Work out the finished part from the listing and answer in its coordinate system (mm). Face numbers are marked on the shaded views. Give positions to 0.01 mm unless a question says otherwise; leave off trailing zeros. Write each loop counter-clockwise with the first axis right and the second up, starting at its lowest first coordinate (ties: lowest second). Pieces come first, ordered by that corner, then holes. Notation, with made-up numbers: (5.5, 19.5) -> (45.5, 19.5) arc R36 cw to (45.5, 56.5) -> close; hole circle Ø6 at (-20.75, -6.5). An arc over 180 degrees is marked (long way). Use a Markdown table: item, result. Add a question column.
Q1. Each of these flat-tipped pins is pushed along its axis until it touches: pin 1 Ø3 at (x, z) = (0, 0) entering from +Y; pin 2 Ø4.5 at (x, z) = (0, 0.5) entering from -Y; pin 3 Ø1 at (x, y) = (39, 0.5) entering from +Z; pin 4 Ø1 at (y, z) = (1, 24) entering from +X. Where does it stop, or does it pass through?
Q2. Section C-C, the plane z = 30 is taken. Give the vertices of the cut face in (x, y), plus the area to 3 significant figures.
Q3. Consider line 1 (X direction, y = 2.55, z = 0); line 2 (X direction, y = 1.15, z = 0); line 3 (X direction, y = 0.35, z = 0). Determine where each line is inside the solid, lowest interval first.
Q4. Section D-D, the plane x = 94.5 is taken. Give the vertices of the cut face in (y, z), plus the area to 3 significant figures.
Q5. Section B-B, the plane x = 52.5 is taken. Give the vertices of the cut face in (y, z), plus the area to 3 significant figures.
Q6. For a pull along Z with two mould halves and no side action, classify the marked faces 1 and 2 as pulls with the +Z half, pulls with the -Z half, needs draft (parallel to the pull), parting line crosses it, or undercut.
Q7. Section A-A, the plane z = 9.5 is taken. Give the vertices of the cut face in (x, y).
Autodesk Inventor part; units mm, degrees
ref_plane "YZ Plane" through (0, 0, 0) normal (1, 0, 0) x (0, 1, 0)
ref_plane "XZ Plane" through (0, 0, 0) normal (0, 1, 0) x (-1, 0, 0)
ref_plane "XY Plane" through (0, 0, 0) normal (0, 0, 1) x (1, 0, 0)
sketch "Szkic4" plane through (0, 0, 0) normal (0, 1, 0) x (-1, 0, 0)
  circle A0 centre (0, 0) radius 2.1
  line L0 (-3, 3) -> (3, 3)
  line L1 (3, 3) -> (3, -3)
  line L2 (3, -3) -> (-3, -3)
  line L3 (-3, -3) -> (-3, 3)
  line L4 (-3, 3) -> (3, -3) construction
  line L5 (3, 3) -> (-3, -3) construction
  line L6 (0, 0) -> (-4.5962, -4.5962)
  line L7 (0, 0) -> (6.5, 0) construction
  line L8 (0, 0) -> (-4.5962, 4.5962)
  line L9 (0, 0) -> (6.5, 0) construction
  arc A1 (-4.5962, 4.5962) -> (-4.5962, -4.5962) centre (0, 0) ccw construction
  arc A2 (-5.3033, 5.3033) -> (-5.3033, -5.3033) centre (0, 0) ccw
  arc A3 (-3.8891, 3.8891) -> (-3.8891, -3.8891) centre (0, 0) ccw
  arc A4 (-3.8891, 3.8891) -> (-5.3033, 5.3033) centre (-4.5962, 4.5962) ccw
  arc A5 (-5.3033, -5.3033) -> (-3.8891, -3.8891) centre (-4.5962, -4.5962) ccw
  line L10 (0, 0) -> (-7.7, 0)
  line L11 (0, 0) -> (7.7, 0) construction
  line L12 (-7.7, 0) -> (-54.7226, -47.0226)
  line L13 (-54.7226, -47.0226) -> (-101.7452, 0)
  line L14 (-101.7452, 0) -> (-54.7226, 47.0226)
  line L15 (-54.7226, 47.0226) -> (-7.7, 0)
  line L16 (-7.7, 0) -> (58.8, 0) construction
  line L17 (-7.7, 0) -> (-8.7, 0)
  line L18 (-8.7, 0) -> (-54.6619, -45.9619)
  line L19 (-54.6619, -45.9619) -> (-100.6239, 0)
  line L20 (-100.6239, 0) -> (-54.6619, 45.9619)
  line L21 (-54.6619, 45.9619) -> (-8.7, 0)
  line L22 (-8.7, 0) -> (56.3, 0) construction
  arc A6 (-18.4411, -10.7411) -> (0, -3) centre (-13.548, 3.4383) ccw
  arc A7 (0, 3) -> (-18.4411, 10.7411) centre (-13.548, -3.4383) ccw
  point P0 (-18.4411, 10.7411)
  point P1 (0, 3)
  point P2 (-3, 0)
  dimension "d52" = 4.2
  dimension "d53" = 6
  dimension "d54" = 6
  dimension "d55" = 6.5
  dimension "d56" = 135
  dimension "d57" = 6.5
  dimension "d58" = 135
  dimension "d59" = 6.5
  dimension "d60" = 2
  dimension "d61" = 7.7
  dimension "d62" = 180
  dimension "d67" = 66.5
  dimension "d68" = 135
  dimension "d69" = 66.5
  dimension "d70" = 1
  dimension "d71" = 65
  dimension "d72" = 135
  dimension "d73" = 65
  dimension "d74" = 20
  dimension "d75" = 15
extrude "Wyciągnięcie proste4" add sketch "Szkic4" along normal blind 3 contours A0 L8 L0 L1 L2 L6 | A0 L10 L3 L8 | L6 L3 L10 A0 | L8 A4 A2 L10 L15 A7 L0 | L3 L10 A3 L8 | L6 A3 L10 L3 | L2 A6 L12 L10 A2 A5 L6 | L15 L12 L13 L14
extrude "Wyciągnięcie proste5" add sketch "Szkic4" along normal blind 1 contours L18 L19 L20 L21
surface extrude "PowWyciągnięciaProstego2" sketch "Szkic4" along normal blind 5.5 shown no curves A3 A4 A2 A5
fillet "Zaokrąglenie1" radius 3 2 edges at (-3, 1.5, 3) (-3, 1.5, -3)
sketch "Szkic5" plane through (0, 1, 0) normal (0, 1, 0) x (1, 0, 0)
  line L0 (8.7, 0) -> (54.6619, 45.9619)
  line L1 (8.7, 0) -> (100.6239, 0)
  circle A0 centre (54.6619, 0) radius 20
  point P0 (0, 0)
  dimension "d84" = 40
extrude "Wyciągnięcie proste6" cut sketch "Szkic5" against normal blind 10
sketch "Szkic6" plane through (0, 3, 0) normal (0, 1, 0) x (1, 0, 0)
  arc A0 (3.8891, -3.8891) -> (3.8891, 3.8891) centre (0, 0) ccw
  arc A1 (3.8891, -3.8891) -> (5.3033, -5.3033) centre (4.5962, -4.5962) ccw
  arc A2 (5.3033, -5.3033) -> (5.3033, 5.3033) centre (0, 0) ccw
  arc A3 (5.3033, 5.3033) -> (3.8891, 3.8891) centre (4.5962, 4.5962) ccw
  line L0 (0, 0) -> (4.5962, 4.5962)
  circle A4 centre (4.5962, 4.5962) radius 0.9
  circle A5 centre (0, 0) radius 2.1
  circle A6 centre (0, 0) radius 1
  point P0 (0, 0)
  dimension "d87" = 1.8
  dimension "d92" = 2
extrude "Wyciągnięcie proste7" add sketch "Szkic6" against normal blind 1 contours A0 A3 A2 A1 | A4 | A5
extrude "Wyciągnięcie proste8" add sketch "Szkic6" along normal blind 2 contours A4
properties part number "flowerstand"
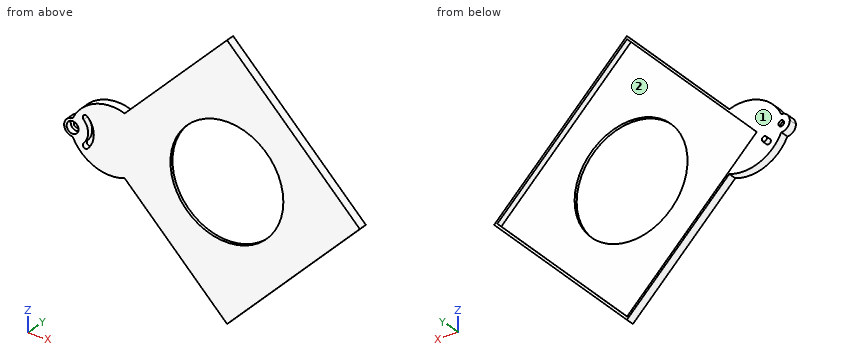
Result set:
| question | item | result |
|---|---|---|
| 1 | pin 1 | stops at y = 3 |
| 1 | pin 2 | stops at y = 0 |
| 1 | pin 3 | stops at z = 31.8 |
| 1 | pin 4 | stops at x = 78.25 |
| 2 | outline | (37.7, 0) -> (71.75, 0) -> (71.75, 3) -> (70.62, 3) -> (70.62, 1) -> (38.7, 1) -> (38.7, 3) -> (37.7, 3) -> close |
| 2 | area | 38.3 mm2 |
| 3 | line 1 | x = -3 to -1, 1 to 8.7, 100.62 to 101.75 |
| 3 | line 2 | x = -3 to -2.1, 2.1 to 5.5, 7.5 to 8.7, 100.62 to 101.75 |
| 3 | line 3 | x = -3 to -2.1, 2.1 to 5.5, 7.5 to 34.66, 74.66 to 101.75 |
| 4 | outline | (0, -7.25) -> (3, -7.25) -> (3, -6.12) -> (1, -6.12) -> (1, 6.12) -> (3, 6.12) -> (3, 7.25) -> (0, 7.25) -> close |
| 4 | area | 19.0 mm2 |
| 5 | outline | (0, -44.8) -> (3, -44.8) -> (3, -43.8) -> (1, -43.8) -> (1, -19.88) -> (0, -19.88) -> close; (0, 19.88) -> (1, 19.88) -> (1, 43.8) -> (3, 43.8) -> (3, 44.8) -> (0, 44.8) -> close |
| 5 | area | 53.8 mm2 |
| 6 | face 1 | needs draft |
| 6 | face 2 | undercut |
| 7 | outline | (5.96, 0) -> (37.06, 0) -> (37.06, 1) -> (18.2, 1) -> (18.2, 3) -> (5.96, 3) -> close; (72.26, 0) -> (92.25, 0) -> (92.25, 3) -> (91.12, 3) -> (91.12, 1) -> (72.26, 1) -> close |
